Geometry check sheet. Reference: the model listing, model coordinates, mm. A direction names the side the tool comes from. Coordinates: 2 decimals unless noted, no trailing zeros. Write each loop counter-clockwise with the first axis right and the second up, starting at its lowest first coordinate (ties: lowest second). Pieces come first, ordered by that corner, then holes. Notation, with made-up numbers: (12, 81) -> (50, 81) arc R15 ccw to (50, 110) -> close; hole circle Ø3 at (16.5, -39). An arc over 180 degrees is marked (long way). Put each result on its own line as item: value. Start each with the question number.
from build123d import *

# Parameters (mm, degrees)
SKETCH_1_W          = 12.3
SKETCH_1_H          = 11.3
EXTRUDE_1_DEPTH     = 2.5
SKETCH_2_W          = 1.5
SKETCH_2_H          = 11.3
EXTRUDE_2_DEPTH     = 4.35
SKETCH_5_W          = 9.3
SKETCH_5_H          = 11.5
CUT_EXTRUDE_1_DEPTH = 1
SKETCH_8_W          = 1.6
SKETCH_8_H          = 11.3
EXTRUDE_5_DEPTH     = 0.7
SKETCH_9_W          = 1.6
SKETCH_9_H          = 11.3
EXTRUDE_6_DEPTH     = 0.7
FILLET_8_R          = 0.3
SKETCH_11_W         = 12.3
SKETCH_11_H         = 5.35
CUT_EXTRUDE_2_DEPTH = 2
SKETCH_12_W         = 12.3
SKETCH_12_H         = 5.35
CUT_EXTRUDE_3_DEPTH = 2
SKETCH_13_W         = 1.5
SKETCH_13_H         = 11.3
EXTRUDE_7_DEPTH     = 0.5
SKETCH_14_W         = 1.5
SKETCH_14_H         = 11.3
EXTRUDE_8_DEPTH     = 0.5
FILLET_9_R          = 0.5
FILLET_10_R         = 0.7


with BuildPart() as part:
    # 스케치1 → 보스-돌출1 (new body)
    with BuildSketch(Plane.XY):
        Rectangle(SKETCH_1_W, SKETCH_1_H)
    extrude(amount=EXTRUDE_1_DEPTH)

    # 스케치2 → 보스-돌출2 (add)
    with BuildSketch(Plane.XY.offset(2.5)):
        with Locations((-5.4, 0)):
            Rectangle(SKETCH_2_W, SKETCH_2_H)
        with Locations((5.4, 0)):
            Rectangle(SKETCH_2_W, SKETCH_2_H)
    extrude(amount=EXTRUDE_2_DEPTH)

    # 스케치5 → 컷-돌출1 (cut)
    with BuildSketch(Plane.XY.offset(2.5)):
        Rectangle(SKETCH_5_W, SKETCH_5_H)
    extrude(amount=-CUT_EXTRUDE_1_DEPTH, mode=Mode.SUBTRACT)

    # 스케치8 → 보스-돌출5 (add)
    with BuildSketch(Plane(origin=(-4.65, 0, 0), x_dir=(0, 0, -1), z_dir=(1, 0, 0))):
        with Locations((-6.05, 0)):
            Rectangle(SKETCH_8_W, SKETCH_8_H)
    extrude(amount=EXTRUDE_5_DEPTH)

    # 스케치9 → 보스-돌출6 (add)
    with BuildSketch(Plane.ZY.offset(-4.65)):
        with Locations((6.05, 0)):
            Rectangle(SKETCH_9_W, SKETCH_9_H)
    extrude(amount=EXTRUDE_6_DEPTH)

    # 필렛8
    fillet_8_edges = [part.edges().sort_by_distance(p)[0] for p in [
        (4.65, 0, 1.5),
        (-4.65, 0, 1.5),
    ]]
    fillet(fillet_8_edges, radius=FILLET_8_R)

    # 스케치11 → 컷-돌출2 (cut)
    with BuildSketch(Plane(origin=(0, 5.65, 0), x_dir=(1, 0, 0), z_dir=(0, 1, 0))):
        with Locations((0, -4.175)):
            Rectangle(SKETCH_11_W, SKETCH_11_H)
    extrude(amount=-CUT_EXTRUDE_2_DEPTH, mode=Mode.SUBTRACT)

    # 스케치12 → 컷-돌출3 (cut)
    with BuildSketch(Plane.XZ.offset(5.65)):
        with Locations((0, 4.175)):
            Rectangle(SKETCH_12_W, SKETCH_12_H)
    extrude(amount=-CUT_EXTRUDE_3_DEPTH, mode=Mode.SUBTRACT)

    # 스케치13 → 보스-돌출7 (add)
    with BuildSketch(Plane(origin=(6.15, 0, 0), x_dir=(0, 0, -1), z_dir=(1, 0, 0))):
        with Locations((-0.75, 0)):
            Rectangle(SKETCH_13_W, SKETCH_13_H)
    extrude(amount=EXTRUDE_7_DEPTH)

    # 스케치14 → 보스-돌출8 (add)
    with BuildSketch(Plane.ZY.offset(6.15)):
        with Locations((0.75, 0)):
            Rectangle(SKETCH_14_W, SKETCH_14_H)
    extrude(amount=EXTRUDE_8_DEPTH)

    # 필렛9
    fillet_9_edges = [part.edges().sort_by_distance(p)[0] for p in [
        (6.15, 0, 1.5),
        (-6.15, 0, 1.5),
    ]]
    fillet(fillet_9_edges, radius=FILLET_9_R - 0.0001)  # a hair under: the kernel refuses the full size

    # 필렛10
    fillet_10_edges = [part.edges().sort_by_distance(p)[0] for p in [
        (-3.95, 0, 6.85),
        (-3.95, 0, 5.25),
        (3.95, 0, 5.25),
        (3.95, 0, 6.85),
    ]]
    fillet(fillet_10_edges, radius=FILLET_10_R - 0.0001)  # a hair under: the kernel refuses the full size


solid = part.part
Item 1: Section check B-B, the plane x = 5.25. Enter the section's corners in (y, z).
Item 2: Section check A-A, the plane z = 3. Enter the section's corners in (x, y), and give its area (3 significant figures).
Item 3: Mould release check, pull along Z, two halves, no side actions. Record for faces 4 (the flat face through (-4.65, 0, 4)), 5 (the flat face through (6.65, 0, 1)), 6 (the flat face through (-5, 0, 6.85)): released by +Z, released by -Z, zero draft, split by the parting line, or undercut.
Item 4: Go/stop test with flat-tipped pins: P1, Ø0.8, axis at x = 5.5, z = 5, coming from the -Y side; P2, Ø1.5, axis at y = 0, z = 4.5, coming from the -X side; P3, Ø1, axis at x = -1.5, y = -2.5, coming from the +Z side. Record where each tip stops, or that it passes through.
Item 5: Scan lines: line 1 along X through (y, z) = (3, 3.75); line 2 along Z through (x, y) = (-2, 3); line 3 along X through (y, z) = (0.5, 6.5). Record each from-to range of solid material in increasing order. Write a range as [from, to].
Item 6: Section check D-D, the plane z = 5.5. Enter the section's corners in (x, y), and give its area (3 significant figures).
Item 7: Access from +Z, -Z, +X, -X, +Y, -Y to the whole of each face (thin tool, end or side, straight path). Record for faces 1 (the flat face through (4.65, 0, 4)), 2 (the flat face through (5, 3.65, 4)), 3 (the flat face through (6.15, 0, 4)).
From the geometry:
1. outline: (-5.65, 0) -> (5.65, 0) -> (5.65, 1.5) -> (3.65, 1.5) -> (3.65, 6.85) -> (-3.65, 6.85) -> (-3.65, 1.5) -> (-5.65, 1.5) -> close
2. outline: (-6.15, -3.65) -> (-4.65, -3.65) -> (-4.65, 3.65) -> (-6.15, 3.65) -> close; (4.65, -3.65) -> (6.15, -3.65) -> (6.15, 3.65) -> (4.65, 3.65) -> close
2. area: 21.9 mm²
3. face 4: undercut
3. face 5: zero draft
3. face 6: released by +Z
4. P1: y = -3.65
4. P2: x = -6.15
4. P3: z = 1.5
5. line 1: [-6.15, -4.65], [4.65, 6.15]
5. line 2: [0, 1.5]
5. line 3: [-6.15, -4.04], [4.04, 6.15]
6. outline: (-6.15, -3.65) -> (-4.11, -3.65) -> (-4.11, 3.65) -> (-6.15, 3.65) -> close; (4.11, -3.65) -> (6.15, -3.65) -> (6.15, 3.65) -> (4.11, 3.65) -> close
6. area: 29.7 mm²
7. face 1: +Y, -Y
7. face 2: +Z, +X, -X, +Y
7. face 3: +Z, +X, +Y, -Y
